```python
from build123d import *

# Parameters (mm, degrees)
SKETCH1_W           = 200
SKETCH1_H           = 20
BOSS_EXTRUDE2_DEPTH = 20
SKETCH3_R           = 5
CUT_EXTRUDE1_DEPTH  = 103.46950766
SKETCH4_R           = 5
CUT_EXTRUDE2_DEPTH  = 104.923048454


with BuildPart() as part:
    # Sketch1 → Boss-Extrude2 (new body)
    with BuildSketch(Plane.XY):
        Rectangle(SKETCH1_W, SKETCH1_H)
    extrude(amount=BOSS_EXTRUDE2_DEPTH)

    # Sketch3 → Cut-Extrude1 (cut, through all)
    with BuildSketch(Plane.XY.offset(20)):
        with Locations((-90, 0)):
            Circle(SKETCH3_R)
    extrude(amount=-CUT_EXTRUDE1_DEPTH, mode=Mode.SUBTRACT)

    # Sketch4 → Cut-Extrude2 (cut, through all)
    with BuildSketch(Plane.XZ.offset(10)):
        with Locations(Location((90, 10, 0), (0, 0, 270))):
            Circle(SKETCH4_R)
    extrude(amount=-CUT_EXTRUDE2_DEPTH, mode=Mode.SUBTRACT)


solid = part.part
```
Can you work these out from the model? Positions are in its coordinate system, mm. Round coordinates to 2 decimals unless told otherwise and drop trailing zeros. Order: outer loops, then holes, each group sorted by start corner. A loop starts at its lowest first (then second) coordinate and runs counter-clockwise, first axis right, second up. Notation, with made-up numbers: (73.5, -14.75) -> (115.5, -14.75) arc R4 ccw to (115.5, -10.75) -> close; hole circle Ø2 at (48, 59.5). An arc over 180 degrees is marked (long way). Return JSON: item names as keys, results as strings. Group by question number.
1. If we section it at C-C, the plane x = -90: Write out the boundary of the cut face in (y, z).
2. We'd pull the mould along Y, two halves only. Please class faces 1 (the face through (-85.381, -1.915, 10.14)), 2 (the face through (-1, 0, 20)), 3 (the face through (-1, -10, 10)): released by +Y, released by -Y, zero draft, split by the parting line, or undercut.
3. I need wall thicknesses on line 1 (Y direction, x = -90, z = 12); line 2 (X direction, y = 0.5, z = 17.5); line 3 (X direction, y = 1, z = 10). Which ranges of each line are inside material? Lowest first, please. Write a range as [from, to].
4. If we section it at A-A, the plane z = 10: Write out the boundary of the cut face in (x, y).
5. If we section it at D-D, the plane z = 2: Write out the boundary of the cut face in (x, y).
6. Will this pin go through, and if not, where does the flat tip stop? pin 1 (8 mm diameter, centred on x = -90, y = 0, fed in from -Z).
7. If we section it at B-B, the plane y = 0: Write out the boundary of the cut face in (x, z).
Output values:
{
 "1": {"outline": "(-10, 0) -> (-5, 0) -> (-5, 20) -> (-10, 20) -> close; (5, 0) -> (10, 0) -> (10, 20) -> (5, 20) -> close"},
 "2": {"face 1": "undercut", "face 2": "zero draft", "face 3": "released by -Y"},
 "3": {"line 1": "[-10, -5], [5, 10]", "line 2": "[-100, -94.97], [-85.03, 100]", "line 3": "[-100, -94.9], [-85.1, 85], [95, 100]"},
 "4": {"outline": "(-100, -10) -> (85, -10) -> (85, 10) -> (-100, 10) -> close; (95, -10) -> (100, -10) -> (100, 10) -> (95, 10) -> close; hole circle Ø10 at (-90, 0)"},
 "5": {"outline": "(-100, -10) -> (100, -10) -> (100, 10) -> (-100, 10) -> close; hole circle Ø10 at (-90, 0)"},
 "6": {"pin 1": "through"},
 "7": {"outline": "(-100, 0) -> (-95, 0) -> (-95, 20) -> (-100, 20) -> close; (-85, 0) -> (100, 0) -> (100, 20) -> (-85, 20) -> close; hole circle Ø10 at (90, 10)"}
}
